Input: dimensioned drawing with shaded views. Units: mm. Origin: part minimum x, y, z. Round coordinates to 2 decimals unless told otherwise and drop trailing zeros. Order: outer loops, then holes, each group sorted by start corner. A loop starts at its lowest first (then second) coordinate and runs counter-clockwise, first axis right, second up. Notation, with made-up numbers: (70, 36) - (87, 36) arc R35 cw to (87, 69) - close; hole circle Ø1 at (88.5, 78). An arc over 180 degrees is marked (long way). Put each result on its own line as item: value. Start each with the question number.
(1) Pin query (flat end, axial travel): P1, Ø8, axis at x = 17, z = 131.5, coming from the -Y side; P2, Ø1, axis at x = 60.5, y = 89, coming from the +Z side. Return the tip coordinate at first contact, or that it passes through.
(2) Section B-B (z = 138.5). Output: boundary loops of the cut face in (x, y).
(3) Material intervals for L1, parallel to Y at x = 18, z = 105; L2, parallel to Y at x = 140, z = 91; L3, parallel to Z at x = 55, y = 84, sorted ascending. Write a range as [from, to].
(4) Section C-C (y = 11.5). Output: boundary loops of the cut face in (x, z).
(5) Section A-A (x = 39). Output: boundary loops of the cut face in (y, z).
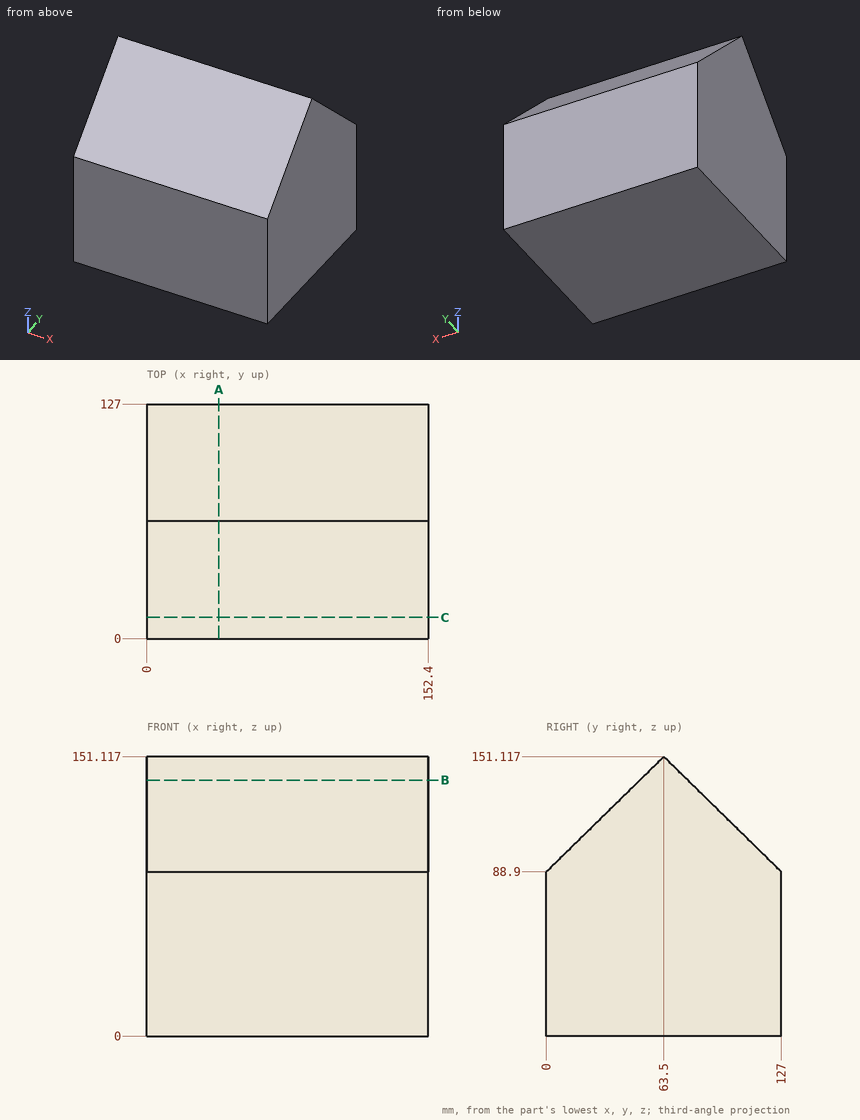
Checks:
1. P1: stops at y = 39.4
1. P2: stops at z = 126.62
2. outline: (0, 50.62) - (152.4, 50.62) - (152.4, 76.38) - (0, 76.38) - close
3. L1: y = [16.43, 110.57]
3. L2: y = [2.14, 124.86]
3. L3: z = [0, 131.03]
4. outline: (0, 0) - (152.4, 0) - (152.4, 100.17) - (0, 100.17) - close
5. outline: (0, 0) - (127, 0) - (127, 88.9) - (63.5, 151.12) - (0, 88.9) - close
